Source: CAD feature listing. Evaluate the final solid. Frame: model axes, mm. Face numbers are marked on the shaded views. A direction names the side the tool comes from. Give positions to 0.01 mm unless a question says otherwise; leave off trailing zeros. Loops run counter-clockwise (first coordinate to the right, second up) from the corner with the lowest first, then second, coordinate; pieces in that order, holes last. Notation, with made-up numbers: M -29,-22 L 1,-22 A10 ccw 1,-16 Z; hole C 69.25,36 d9. An arc over 180 degrees is marked long. Write item = value, one per line.
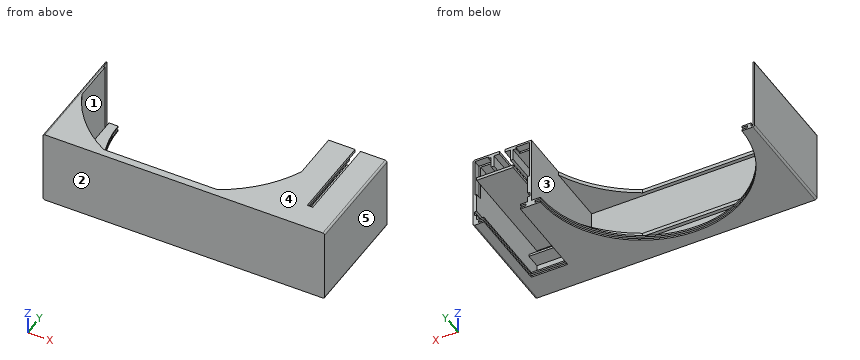
from build123d import *

# Parameters (mm, degrees)
ESQUISSE1_W              = 154.4
ESQUISSE1_H              = 40.8
BOSS_EXTRU_1_DEPTH       = 2
ESQUISSE2_W              = 154.4
ESQUISSE2_H              = 40.8
ESQUISSE2_W_2            = 120.4
ESQUISSE2_H_2            = 8.4
ESQUISSE2_H_3            = 25.4
BOSS_EXTRU_2_DEPTH       = 60.2
ENL_V_MAT_EXTRU_1_REACH  = 173.385
ESQUISSE4_W              = 1
ESQUISSE4_H              = 39.8
ENL_V_MAT_EXTRU_2_DEPTH  = 4
ESQUISSE5_W              = 1.2
ESQUISSE5_H              = 2.4
ENL_V_MAT_EXTRU_3_DEPTH  = 20.2
BOSS_EXTRU_3_DEPTH       = 8
ESQUISSE9_W              = 9
ESQUISSE9_H              = 51.7
ENL_V_MAT_EXTRU_5_DEPTH  = 6.4
ESQUISSE10_W             = 3
ESQUISSE10_H             = 47.7
ENL_V_MAT_EXTRU_6_DEPTH  = 172.011227702
ESQUISSE11_W             = 20
ESQUISSE11_H             = 1.6
BOSS_EXTRU_4_DEPTH       = 60.2
ENL_V_MAT_EXTRU_7_REACH  = 173.385
ESQUISSE12_R             = 55.2
ENL_V_START              = -0.9
ESQUISSE14_R             = 58.2
ENL_V_MAT_EXTRU_8_DEPTH  = 1.2
CONG_1_R                 = 1
ENL_V_MAT_EXTRU_9_REACH  = 173.385
ESQUISSE15_W             = 20
ESQUISSE15_H             = 47.2
ESQUISSE16_W             = 26
ESQUISSE16_H             = 53.2
ESQUISSE16_W_2           = 20
ESQUISSE16_H_2           = 47.2
ENL_V_MAT_EXTRU_11_DEPTH = 1.2


with BuildPart() as part:
    # Esquisse1 → Boss.-Extru.1 (new body)
    with BuildSketch(Plane(origin=(0, 0, 0), x_dir=(1, 0, 0), z_dir=(0, 1, 0))):
        with Locations((77.2, 20.4)):
            Rectangle(ESQUISSE1_W, ESQUISSE1_H)
    extrude(amount=BOSS_EXTRU_1_DEPTH)

    # Esquisse2 → Boss.-Extru.2 (add)
    with BuildSketch(Plane(origin=(0, 2, 0), x_dir=(1, 0, 0), z_dir=(0, 1, 0))):
        with Locations((77.2, 20.4)):
            Rectangle(ESQUISSE2_W, ESQUISSE2_H)
        with Locations((62.2, 33.6)):
            Rectangle(ESQUISSE2_W_2, ESQUISSE2_H_2, mode=Mode.SUBTRACT)
        with Locations((62.2, 14.7)):
            Rectangle(ESQUISSE2_W_2, ESQUISSE2_H_3, mode=Mode.SUBTRACT)
        Polygon((124.4, 37.8), (124.4, 2), (132.4, 2), (132.4, 8), (144.4, 8), (144.4, 2), (152.4, 2), (152.4, 37.8), align=None, mode=Mode.SUBTRACT)
    extrude(amount=BOSS_EXTRU_2_DEPTH)

    # Enlèv. mat.-Extru.1: up to this face of the body (flat: up to its plane)
    enl_v_mat_extru_1_end = Plane(part.part.faces().sort_by_distance((62.2, 32.1, -29.4))[0])
    # Esquisse3 → Enlèv. mat.-Extru.1 (cut, up to the picked face)
    with BuildSketch(Plane.XY, mode=Mode.PRIVATE) as enl_v_mat_extru_1_sk1:
        with BuildLine():
            Line((2, 62.2), (122.4, 62.2))
            Line((122.4, 62.2), (122.4, 35.145240714))
            ThreePointArc((122.4, 35.145240714), (110.444857601, 17.16186377), (93.324909638, 4))
            Line((93.324909638, 4), (31.075090362, 4))
            ThreePointArc((31.075090362, 4), (13.955142399, 17.16186377), (2, 35.145240714))
            Line((2, 35.145240714), (2, 62.2))
        make_face()
    enl_v_mat_extru_1_tool1 = split(extrude(enl_v_mat_extru_1_sk1.sketch, amount=-ENL_V_MAT_EXTRU_1_REACH, mode=Mode.PRIVATE), bisect_by=enl_v_mat_extru_1_end, keep=Keep.BOTH, mode=Mode.PRIVATE)
    add(enl_v_mat_extru_1_tool1.solids().sort_by(Axis((62.2, 35.325026, 0), (0, 0, -1)))[0], mode=Mode.SUBTRACT)

    # Esquisse4 → Enlèv. mat.-Extru.2 (cut)
    with BuildSketch(Plane(origin=(0, 62.2, 0), x_dir=(1, 0, 0), z_dir=(0, 1, 0))):
        with Locations((1.5, 19.9)):
            Rectangle(ESQUISSE4_W, ESQUISSE4_H)
        Polygon((130.9, 1), (130.9, 2), (124.4, 2), (124.4, 22), (123.4, 22), (123.4, 2), (123.4, 1), align=None)
        Polygon((152.4, 2), (152.4, 22), (153.4, 22), (153.4, 2), (153.4, 1), (145.9, 1), (145.9, 2), align=None)
    extrude(amount=-ENL_V_MAT_EXTRU_2_DEPTH, mode=Mode.SUBTRACT)

    # Esquisse5 → Enlèv. mat.-Extru.3 (cut)
    with BuildSketch(Plane(origin=(0, 62.2, 0), x_dir=(1, 0, 0), z_dir=(0, 1, 0))):
        with Locations((123.8, 33.6)):
            Rectangle(ESQUISSE5_W, ESQUISSE5_H)
        with Locations((153, 33.6)):
            Rectangle(ESQUISSE5_W, ESQUISSE5_H)
    extrude(amount=-ENL_V_MAT_EXTRU_3_DEPTH, mode=Mode.SUBTRACT)

    # Esquisse6 → Boss.-Extru.3 (add)
    with BuildSketch(Plane(origin=(0, 2, 0), x_dir=(1, 0, 0), z_dir=(0, 1, 0))):
        Polygon((133, 22.4), (133, 37.8), (131.8, 37.8), (131.8, 21.2), (152.4, 21.2), (152.4, 22.4), align=None)
    extrude(amount=BOSS_EXTRU_3_DEPTH)

    # Esquisse9 → Enlèv. mat.-Extru.5 (cut)
    with BuildSketch(Plane(origin=(0, 0, -8), x_dir=(-1, 0, 0), z_dir=(0, 0, -1))):
        with Locations((-138.4, 36.35)):
            Rectangle(ESQUISSE9_W, ESQUISSE9_H)
    extrude(amount=-ENL_V_MAT_EXTRU_5_DEPTH, mode=Mode.SUBTRACT)

    # Esquisse10 → Enlèv. mat.-Extru.6 (cut, through all)
    with BuildSketch(Plane(origin=(0, 0, -1.6), x_dir=(-1, 0, 0), z_dir=(0, 0, -1))):
        with Locations((-138.4, 38.35)):
            Rectangle(ESQUISSE10_W, ESQUISSE10_H)
    extrude(amount=-ENL_V_MAT_EXTRU_6_DEPTH, mode=Mode.SUBTRACT)

    # Esquisse11 → Boss.-Extru.4 (add)
    with BuildSketch(Plane(origin=(0, 2, 0), x_dir=(1, 0, 0), z_dir=(0, 1, 0))):
        with Locations((142.4, 12.3)):
            Rectangle(ESQUISSE11_W, ESQUISSE11_H)
    extrude(amount=BOSS_EXTRU_4_DEPTH)

    # Esquisse12 → Enlèv. mat.-Extru.7 (cut, up to next)
    with BuildSketch(Plane(origin=(0, 0, -40.8), x_dir=(-1, 0, 0), z_dir=(0, 0, -1)), mode=Mode.PRIVATE) as enl_v_mat_extru_7_sk1:
        with Locations((-62.2, 62.2)):
            Circle(ESQUISSE12_R)
    enl_v_mat_extru_7_tool1 = extrude(enl_v_mat_extru_7_sk1.sketch, amount=-ENL_V_MAT_EXTRU_7_REACH, mode=Mode.PRIVATE) & part.part
    add(enl_v_mat_extru_7_tool1.solids().sort_by_distance((62.2, 62.2, -40.8))[0], mode=Mode.SUBTRACT)

    # Esquisse14 → Enlèv. mat.-Extru.8 (cut)
    with BuildSketch(Plane(origin=(0, 0, -40.8), x_dir=(-1, 0, 0), z_dir=(0, 0, -1)).offset(ENL_V_START)):
        with Locations((-62.2, 62.2)):
            Circle(ESQUISSE14_R)
    extrude(amount=-ENL_V_MAT_EXTRU_8_DEPTH, mode=Mode.SUBTRACT)

    # Congé1
    cong_1_edges = [part.edges().sort_by_distance(p)[0] for p in [
        (0, 31.1, -40.8),
        (154.4, 31.1, -40.8),
        (154.4, 31.1, 0),
        (0, 31.1, 0),
    ]]
    fillet(cong_1_edges, radius=CONG_1_R - 0.0001)  # a hair under: the kernel refuses the full size

    # Esquisse15 → Enlèv. mat.-Extru.9 (cut, up to next)
    with BuildSketch(Plane(origin=(0, 0, -40.8), x_dir=(-1, 0, 0), z_dir=(0, 0, -1)), mode=Mode.PRIVATE) as enl_v_mat_extru_9_sk1:
        with Locations((-138.4, 38.6)):
            Rectangle(ESQUISSE15_W, ESQUISSE15_H)
    enl_v_mat_extru_9_tool1 = extrude(enl_v_mat_extru_9_sk1.sketch, amount=-ENL_V_MAT_EXTRU_9_REACH, mode=Mode.PRIVATE) & part.part
    add(enl_v_mat_extru_9_tool1.solids().sort_by_distance((138.4, 38.6, -40.8))[0], mode=Mode.SUBTRACT)

    # Esquisse16 → Enlèv. mat.-Extru.11 (cut)
    with BuildSketch(Plane(origin=(0, 0, -40.8), x_dir=(-1, 0, 0), z_dir=(0, 0, -1)).offset(ENL_V_START)):
        with Locations((-138.4, 38.6)):
            Rectangle(ESQUISSE16_W, ESQUISSE16_H)
        with Locations((-138.4, 38.6)):
            Rectangle(ESQUISSE16_W_2, ESQUISSE16_H_2, mode=Mode.SUBTRACT)
    extrude(amount=-ENL_V_MAT_EXTRU_11_DEPTH, mode=Mode.SUBTRACT)


solid = part.part
1. Pull-direction query (Z, two-part tool) for the marked faces 3, 4 and 5; classes: +Z half, -Z half, draft (parallel to the pull), parting line (faces both ways), or undercut.
Derived:
face_3 = undercut
face_4 = +Z half
face_5 = draft
2. First-contact query: pin 1 Ø0.5 at (x, y) = (1.5, 60.5) entering from +Z; pin 2 Ø1.5 at (x, z) = (66, -31.5) entering from +Y; pin 3 Ø3 at (x, z) = (139, -4.5) entering from +Y; pin 4 Ø1.5 at (x, z) = (107, -25.5) entering from -Y. Flat tips, straight axial feed; report the tip coordinate or a pass-through.
Derived:
pin_1 = -39.8
pin_2 = 2
pin_3 = 10.5
pin_4 = 0
3. Cut plane C-C, the plane y = 37. Count the separate pieces of the cut face and the enclosed holes in it, then the cut area to 3 significant figures.
Derived:
separate_pieces = 3
enclosed_holes = 0
area = 417 mm²
4. Reachability of the marked faces 1 and 2 from +Z, -Z, +X, -X, +Y, -Y: full face, straight path, thin tool, end or side. Return the list, or none.
Derived:
face_1 = +Y
face_2 = +Z, -Z, +X, -X, -Y
5. Cut plane B-B, the plane x = 62.2. Return the cut outline in (y, z).
Derived:
outline = M 0,-40.8 L 7,-40.8 L 7,-39.9 L 4,-39.9 L 4,-38.7 L 7,-38.7 L 7,-37.8 L 2,-37.8 L 2,-29.4 L 4,-29.4 L 4,-27.4 L 2,-27.4 L 2,-2 L 4,-2 L 4,0 L 0,0 Z
6. Cut plane D-D, the plane x = 42. Return the cut outline in (y, z), then the cut area to 3 significant figures.
Derived:
outline = M 0,-40.8 L 10.83,-40.8 L 10.83,-39.9 L 7.62,-39.9 L 7.62,-38.7 L 10.83,-38.7 L 10.83,-37.8 L 2,-37.8 L 2,-29.4 L 4,-29.4 L 4,-27.4 L 2,-27.4 L 2,-2 L 4,-2 L 4,0 L 0,0 Z
area = 112 mm²
7. Cut plane A-A, the plane z = -10. Return the cut outline in (x, y), then the cut area to 3 significant figures.
Derived:
outline = M 0,0 L 154.4,0 L 154.4,62.2 L 153.4,62.2 L 153.4,58.2 L 152.4,58.2 L 152.4,2 L 124.4,2 L 124.4,58.2 L 123.4,58.2 L 123.4,62.2 L 122.4,62.2 L 122.4,2 L 2,2 L 2,58.2 L 1,58.2 L 1,62.2 L 0,62.2 Z
area = 658 mm²
8. Material intervals for probe 1 along X at (y, z) = (38.5, -18); probe 2 along X at (y, z) = (48.5, -4); probe 3 along X at (y, z) = (44, -33), sorted ascending. Write a range as from..to.
Derived:
probe_1 = 0..2, 122.4..124.4, 152.4..154.4
probe_2 = 0..2, 122.4..124.4, 132.4..133.9, 142.9..144.4, 152.4..154.4
probe_3 = 0..2, 122.4..123.2, 153.6..154.4
